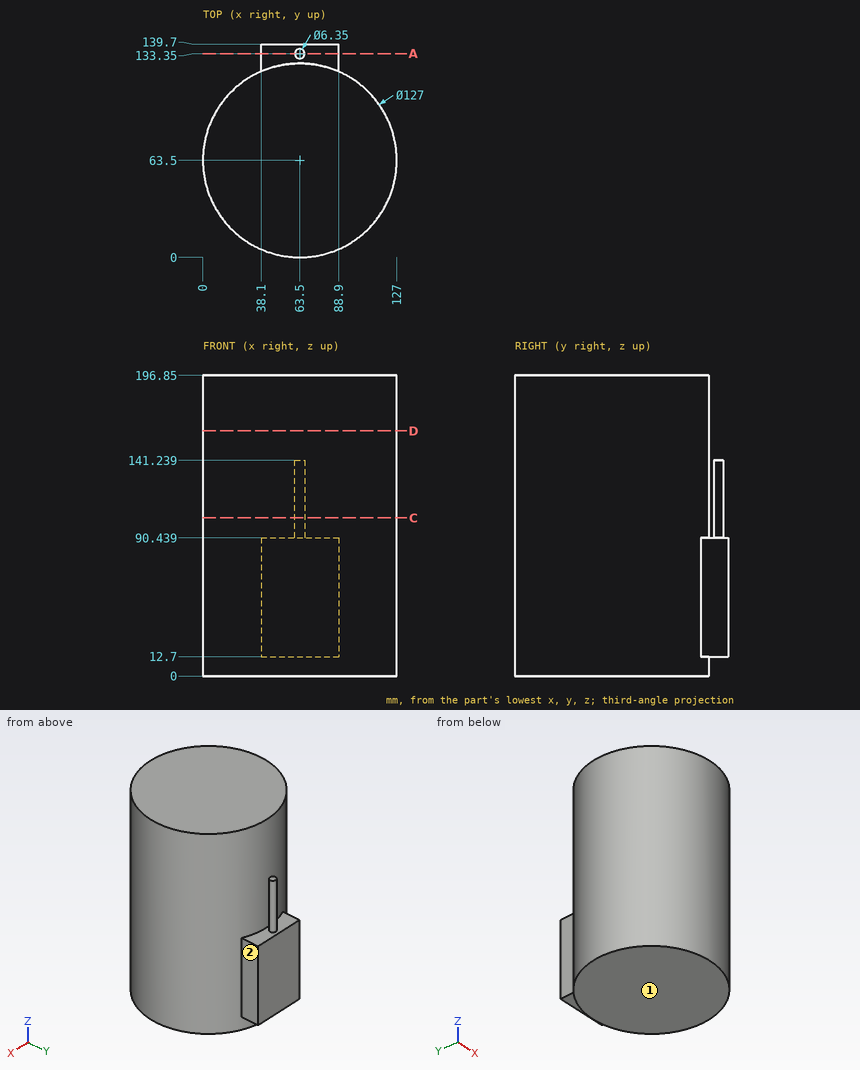
Here's the drawing with two shaded views (mm, measured from the low corner). I have some questions. A direction names the side the tool comes from. Coordinates: 2 decimals unless noted, no trailing zeros. Order: outer loops, then holes, each group sorted by start corner. A loop starts at its lowest first (then second) coordinate and runs counter-clockwise, first axis right, second up. Notation, with made-up numbers: (41.5, 73) - (65.5, 73) arc R15 ccw to (65.5, 79) - close; hole circle Ø5 at (-18.5, 42). An arc over 180 degrees is marked (long way). Answer in a Markdown table with one row per item. Add a question column.
(1) If we section it at D-D, the plane z = 160.5: Please give me the cut outline in (x, y), then the cut area to 3 significant figures.
(2) If we section it at A-A, the plane y = 133.35: Please give me the cut outline in (x, z) (1 decimal).
(3) If we section it at C-C, the plane z = 103.5: Please give me the cut outline in (x, y) (3 decimals).
(4) I need wall thicknesses on L1, parallel to Z at x = 39.5, y = 134; L2, parallel to Y at x = 81, z = 43; L3, parallel to X at y = 104.5, z = 32.5. Which ranges of each line are inside material? Lowest first, please.
(5) Will these pins go through, and if not, where does the flat tip stop? pin 1 (20 mm diameter, centred on y = 132, z = 42, fed in from -X); pin 2 (8 mm diameter, centred on y = 36.5, z = 38, fed in from +X); pin 3 (20 mm diameter, centred on y = 130.5, z = 53.5, fed in from +X) (1 decimal).
(6) On a 3-axis mill with a long thin cutter (end or side, diameter ignored), from which of +Z, -Z, +X, -X, +Y, -Y can I reach the whole of each face in a straight line? I mean the marked faces 1 and 2. Say none if no direction works.
Results are:
| question | item | result |
|---|---|---|
| 1 | outline | circle Ø127 at (63.5, 63.5) |
| 1 | area | 12,700 mm2 |
| 2 | outline | (38.1, 12.7) - (88.9, 12.7) - (88.9, 90.4) - (66.7, 90.4) - (66.7, 141.2) - (60.3, 141.2) - (60.3, 90.4) - (38.1, 90.4) - close |
| 3 | outline | circle Ø127 at (63.5, 63.5); circle Ø6.35 at (63.5, 133.35) |
| 4 | L1 | z = 12.7 to 90.44 |
| 4 | L2 | y = 2.46 to 139.7 |
| 4 | L3 | x = 15.01 to 111.99 |
| 5 | pin 1 | stops at x = 38.1 |
| 5 | pin 2 | stops at x = 122.69 |
| 5 | pin 3 | stops at x = 91.5 |
| 6 | face 1 | -Z, +X, -X, +Y, -Y |
| 6 | face 2 | +Z, -Z, +X, +Y |
